from build123d import *

# Parameters (mm, degrees)
SKETCH1_R           = 2.5
BOSS_EXTRUDE1_DEPTH = 3
CUT_EXTRUDE1_DEPTH  = 238.479604387


with BuildPart() as part:
    # Sketch1 → Boss-Extrude1 (new body)
    with BuildSketch(Plane(origin=(0, 0, 0), x_dir=(1, 0, 0), z_dir=(0, 1, 0))):
        with BuildLine():
            Line((-227.25, 10), (227.25, 10))
            ThreePointArc((227.25, 10), (237.25, 0), (227.25, -10))
            Line((227.25, -10), (-227.25, -10))
            ThreePointArc((-227.25, -10), (-237.25, 0), (-227.25, 10))
        make_face()
        with Locations(Location((-227.25, 0, 0), (0, 0, 270))):
            Circle(SKETCH1_R, mode=Mode.SUBTRACT)
        with BuildLine():
            Line((230.25, -2.5), (220.25, -2.5))
            ThreePointArc((220.25, -2.5), (217.75, 0), (220.25, 2.5))
            Line((220.25, 2.5), (230.25, 2.5))
            ThreePointArc((230.25, 2.5), (232.75, 0), (230.25, -2.5))
        make_face(mode=Mode.SUBTRACT)
    extrude(amount=BOSS_EXTRUDE1_DEPTH)

    # Sketch2 → Cut-Extrude1 (cut, through all)
    with BuildSketch(Plane(origin=(0, 3, 0), x_dir=(1, 0, 0), z_dir=(0, 1, 0))):
        with BuildLine():
            Line((-127.25, 2.5), (22.75, 2.5))
            ThreePointArc((22.75, 2.5), (25.25, 0), (22.75, -2.5))
            Line((22.75, -2.5), (-127.25, -2.5))
            ThreePointArc((-127.25, -2.5), (-129.75, 0), (-127.25, 2.5))
        make_face()
    extrude(amount=-CUT_EXTRUDE1_DEPTH, mode=Mode.SUBTRACT)


solid = part.part
Source: CAD feature listing. Evaluate the final solid. Frame: model axes, mm. Round coordinates to 2 decimals unless told otherwise and drop trailing zeros. Write each loop counter-clockwise with the first axis right and the second up, starting at its lowest first coordinate (ties: lowest second). Pieces come first, ordered by that corner, then holes. Notation, with made-up numbers: M 46.25,67.5 L 76.25,67.5 A35 ccw 76.25,106.5 Z; hole C -8.5,30 d6. An arc over 180 degrees is marked long. One line per item, written item: value. Start each with the question number.
Item 1: Ray query, L1, parallel to X at y = 0.95, z = 0; L2, parallel to Z at x = -103, y = 1.2; L3, parallel to X at y = 1.7, z = 1. Return the intervals inside material, ascending. Write a range as from..to.
Item 2: Section query A-A (y = 1.8). Return the cut outline in (x, z), plus the area to 3 significant figures.
Item 3: Pin query (flat end, axial travel): pin 1 (4.5 mm diameter, centred on x = -227.25, z = 0, fed in from -Y). Return the tip coordinate at first contact, or that it passes through.
Item 4: Section query B-B (x = -59.5). Return the cut outline in (y, z).
Result set:
1. L1: x = -237.25..-229.75, -224.75..-129.75, 25.25..217.75, 232.75..237.25
1. L2: z = -10..-2.5, 2.5..10
1. L3: x = -237.2..-229.54, -224.96..-129.54, 25.04..217.96, 232.54..237.2
2. outline: M -227.25,-10 L 227.25,-10 A10 ccw 227.25,10 L -227.25,10 A10 ccw Z; hole C -227.25,0 d5; hole M -127.25,-2.5 L 22.75,-2.5 A2.5 ccw 22.75,2.5 L -127.25,2.5 A2.5 ccw Z; hole M 220.25,-2.5 L 230.25,-2.5 A2.5 ccw 230.25,2.5 L 220.25,2.5 A2.5 ccw Z
2. area: 8,550 mm²
3. pin 1: passes through
4. outline: M 0,-10 L 3,-10 L 3,-2.5 L 0,-2.5 Z; M 0,2.5 L 3,2.5 L 3,10 L 0,10 Z
